Design review of the part built by this model. Coordinates are the model's own, in mm. A direction names the side the tool comes from. Give positions to 0.01 mm unless a question says otherwise; leave off trailing zeros. Write each loop counter-clockwise with the first axis right and the second up, starting at its lowest first coordinate (ties: lowest second). Pieces come first, ordered by that corner, then holes. Notation, with made-up numbers: (8, -38.75) - (64, -38.75) arc R17 cw to (64, -13.75) - close; hole circle Ø1 at (17, 39). An arc over 180 degrees is marked (long way). Write each question's results on one line, items separated by ' | '. Start each with the question number.
from build123d import *

# Parameters (mm, degrees)
SKETCH1_W           = 46.99
SKETCH1_H           = 9.525
SKETCH1_R           = 1.5875
BOSS_EXTRUDE1_DEPTH = 3.175
SKETCH2_R           = 1.5875
BOSS_EXTRUDE2_DEPTH = 1.5875
SKETCH4_W           = 46.99
SKETCH4_H           = 34.925
SKETCH4_R           = 2.4892
BOSS_EXTRUDE3_DEPTH = 3.175


with BuildPart() as part:
    # Sketch1 → Boss-Extrude1 (new body)
    with BuildSketch(Plane.XY):
        Rectangle(SKETCH1_W, SKETCH1_H)
        with Locations((-16.002, 0)):
            Circle(SKETCH1_R, mode=Mode.SUBTRACT)
        with Locations((16.002, 0)):
            Circle(SKETCH1_R, mode=Mode.SUBTRACT)
    extrude(amount=BOSS_EXTRUDE1_DEPTH)

    # Sketch2 → Boss-Extrude2 (add, symmetric)
    with BuildSketch(Plane(origin=(0, 0, 0), x_dir=(0, 0, -1), z_dir=(1, 0, 0))):
        Polygon((50.8, 17.4625), (0, 4.7625), (0, -4.7625), (50.8, -17.4625), align=None)
        with Locations((9.398, 0)):
            Circle(SKETCH2_R, mode=Mode.SUBTRACT)
        with Locations((41.402, 0)):
            Circle(SKETCH2_R, mode=Mode.SUBTRACT)
    extrude(amount=BOSS_EXTRUDE2_DEPTH, both=True)

    # Sketch4 → Boss-Extrude3 (add)
    with BuildSketch(Plane(origin=(0, 0, -50.8), x_dir=(-1, 0, 0), z_dir=(0, 0, -1))):
        Rectangle(SKETCH4_W, SKETCH4_H)
        with Locations((-14.951363636, 11.1125)):
            Circle(SKETCH4_R, mode=Mode.SUBTRACT)
        with Locations((14.951363636, 11.1125)):
            Circle(SKETCH4_R, mode=Mode.SUBTRACT)
        with Locations((14.951363636, -11.1125)):
            Circle(SKETCH4_R, mode=Mode.SUBTRACT)
        with Locations((-14.951363636, -11.1125)):
            Circle(SKETCH4_R, mode=Mode.SUBTRACT)
    extrude(amount=BOSS_EXTRUDE3_DEPTH)


solid = part.part
Q1. Add section A-A on x = 10. State the section outline as (y, z) points (1 decimal), plus the area to 3 significant figures.
Q2. The part is to be moulded in two halves that separate along Y. For faces 1 (the face through (-14.536, -0.608, 1.565)), 2 (the face through (0, 0, -53.975)), 3 (the face through (0, 17.462, -52)), say which applies: +Y half, -Y half, draft (parallel to the pull), parting line (faces both ways), or undercut.
Q3. Machinability: for faces 4 (the face through (0, -4.762, 2)), 5 (the face through (14.416, 0.07, 1.565)), 6 (the face through (-1.588, 0, -31)), 7 (the face through (13, 0, -50.8)), which of the approach directions +Z, -Z, +X, -X, +Y, -Y give a long, thin tool a straight path to every point of the face, cutting with its end or side? Answer none if there is none.
Q4. Add section B-B on y = 0. State the section outline as (x, z) points (1 decimal), plus the area to 3 significant figures.
Q5. For line 1 along X through (y, z) = (-4, -22); line 2 along Z through (x, y) = (-4, -7) (3 decimals); line 3 along Y through (x, z) = (-3, 0.5), list the stretches that pass through material, from the lowest coordinate up. Write a range as [from, to].
Q6. Add section D-D on z = -18. State the section outline as (x, y) points, plus the area to 3 significant figures.
Q7. Insertion check: P1, Ø10, axis at y = 7, z = -43.5, coming from the -X side; P2, Ø6, axis at y = 12.5, z = -11.5, coming from the +X side; P3, Ø1.6, axis at x = -11.5, z = 2, coming from the -Y side; P4, Ø10.5, axis at y = -8.5, z = -37, coming from the +X side. Each pin has a flat end and moves straight along its axis. Give the tip position at first contact, or say it passes through.
Result:
1) outline: (-17.5, -54) - (17.5, -54) - (17.5, -50.8) - (-17.5, -50.8) - close; (-4.8, 0) - (4.8, 0) - (4.8, 3.2) - (-4.8, 3.2) - close | area: 141 mm²
2) face 1: undercut | face 2: draft | face 3: +Y half
3) face 4: +Z, +X, -X, -Y | face 5: +Z | face 6: -X, +Y, -Y | face 7: +X, +Y, -Y
4) outline: (-23.5, -54) - (23.5, -54) - (23.5, -50.8) - (1.6, -50.8) - (1.6, -43) - (-1.6, -43) - (-1.6, -50.8) - (-23.5, -50.8) - close; (-23.5, 0) - (-17.6, 0) - (-17.6, 3.2) - (-23.5, 3.2) - close; (-14.4, 0) - (-1.6, 0) - (-1.6, -7.8) - (1.6, -7.8) - (1.6, 0) - (14.4, 0) - (14.4, 3.2) - (-14.4, 3.2) - close; (-1.6, -39.8) - (1.6, -39.8) - (1.6, -11) - (-1.6, -11) - close; (17.6, 0) - (23.5, 0) - (23.5, 3.2) - (17.6, 3.2) - close | area: 419 mm²
5) line 1: x = [-1.59, 1.59] | line 2: z = [-53.975, -50.8] | line 3: y = [-4.76, 4.76]
6) outline: (-1.59, -9.26) - (1.59, -9.26) - (1.59, 9.26) - (-1.59, 9.26) - close | area: 58.8 mm²
7) P1: stops at x = -1.59 | P2: passes through | P3: stops at y = -4.76 | P4: stops at x = 1.59
